Check sheet for the modelled part. Datum: model origin and axes. Units: mm. A direction names the side the tool comes from. Round coordinates to 2 decimals unless told otherwise and drop trailing zeros. Write each loop counter-clockwise with the first axis right and the second up, starting at its lowest first coordinate (ties: lowest second). Pieces come first, ordered by that corner, then holes. Notation, with made-up numbers: (-39, -22) - (3, -22) arc R11 ccw to (3, -2) - close; hole circle Ø2 at (35, 26.25). An arc over 180 degrees is marked (long way). Answer as a JSON object with one key per item and string values. Group by question number.
Item 1: Thickness scan on line 1 (Y direction, x = -0.5, z = 13); line 2 (Y direction, x = 31, z = 14.5); line 3 (Y direction, x = 42, z = 2). Record the ranges inside material, lowest first.
Item 2: Sectioned sample at B-B on z = 13.75. Count the separate pieces of the cut face and the enclosed holes in it, plus the area to 3 significant figures.
Item 3: Gauge pin test, flat ends, axial feed: P1, Ø1, axis at y = 29.5, z = 12, coming from the +X side; P2, Ø0.6, axis at x = 16, y = 10.5, coming from the +Z side; P3, Ø4, axis at x = 15.5, y = 42.5, coming from the +Z side. Record the tip position at first contact, or that the pin passes through.
Item 4: Sectioned sample at C-C on x = 3.5. Record the boundary of the cut face in (y, z), plus the area to 3 significant figures.
Item 5: Set-up check for faces 1 (the flat face through (-6, 42.249, 7)), 2 (the flat face through (35, 46.247, 10)), 3 (the flat face through (17.1, 18.4, 2)): record each of +Z, -Z, +X, -X, +Y, -Y from which the full face is reachable in a straight line by a thin tool's end or side.
Item 6: Release check for a two-part mould opening along Y. For faces 4 (the flat face through (16, 62.251, 8)), 5 (the flat face through (-2, -1.747, 10)), 6 (the flat face through (12.48, 21.47, 1.97)), 7 (the flat face through (-13.672, -8, 8)) record: pulls with the +Y half, pulls with the -Y half, needs draft (parallel to the pull), parting line crosses it, or undercut.
Item 7: Sectioned sample at D-D on y = 56.5. Record the boundary of the cut face in (x, z).
Item 8: Sectioned sample at A-A on x = 37.5. Record the boundary of the cut face in (y, z).
```python
from build123d import *

# Parameters (mm, degrees)
SKETCH1_W           = 60.000998497
SKETCH1_H           = 80.001998902
BOSS_EXTRUDE1_DEPTH = 15.001
SKETCH2_W           = 14.999998093
SKETCH2_H           = 39.998000621
CUT_EXTRUDE1_DEPTH  = 80.035391071
SKETCH3_W           = 14.99999988
SKETCH3_H           = 39.998000621
CUT_EXTRUDE2_DEPTH  = 80.035391071
CUT_EXTRUDE3_DEPTH  = 11.003000021
BOSS_EXTRUDE2_DEPTH = 6.004000425
CUT_EXTRUDE4_DEPTH  = 80.035391071
CUT_EXTRUDE5_DEPTH  = 80.035391071
BOSS_EXTRUDE3_DEPTH = 6.004000425
CUT_EXTRUDE6_DEPTH  = 80.035391071
BOSS_EXTRUDE4_DEPTH = 11.003000021
CUT_EXTRUDE7_DEPTH  = 11.003000021
BOSS_EXTRUDE5_DEPTH = 11.003000021
CUT_EXTRUDE8_DEPTH  = 11.003000021


with BuildPart() as part:
    # Sketch1 → Boss-Extrude1 (new body)
    with BuildSketch(Plane.XY.offset(15)):
        with Locations((16.328499318, 22.25)):
            Rectangle(SKETCH1_W, SKETCH1_H)
    extrude(amount=-BOSS_EXTRUDE1_DEPTH)

    # Sketch2 → Cut-Extrude1 (cut, through all)
    with BuildSketch(Plane(origin=(0, 0, -0.001), x_dir=(-1, 0, 0), z_dir=(0, 0, -1))):
        with Locations((-38.82899952, 22.250000239)):
            Rectangle(SKETCH2_W, SKETCH2_H)
    extrude(amount=-CUT_EXTRUDE1_DEPTH, mode=Mode.SUBTRACT)

    # Sketch3 → Cut-Extrude2 (cut, through all)
    with BuildSketch(Plane(origin=(0, 0, -0.001), x_dir=(-1, 0, 0), z_dir=(0, 0, -1))):
        with Locations((6.171999991, 22.250000239)):
            Rectangle(SKETCH3_W, SKETCH3_H)
    extrude(amount=-CUT_EXTRUDE2_DEPTH, mode=Mode.SUBTRACT)

    # Sketch4 → Cut-Extrude3 (cut)
    with BuildSketch(Plane.XY.offset(15)):
        Polygon((27.332000732, 42.25), (27.332000732, 46.247001648), (42.331001282, 46.247001648), (42.331001282, 58.252998352), (-9.673999786, 58.252998352), (-9.673999786, 46.247001648), (5.324999809, 46.247001648), (5.324999809, 42.25), (5.326000214, 42.25), (5.326000214, 2.249000072), (5.324999809, 2.249000072), (5.324999809, -1.746999979), (-9.673999786, -1.746999979), (-9.673999786, -13.753000259), (42.331001282, -13.753000259), (42.331001282, -1.746999979), (27.332000732, -1.746999979), (27.332000732, 2.249000072), (27.330999374, 2.249000072), (27.330999374, 42.25), align=None)
    extrude(amount=-CUT_EXTRUDE3_DEPTH, mode=Mode.SUBTRACT)

    # Sketch5 → Boss-Extrude2 (add)
    with BuildSketch(Plane.XY.offset(3.996999979)):
        Polygon((16.327999115, 4.750999928), (17.579000473, 4.414999962), (18.493999481, 3.5), (18.829000473, 2.25), (18.493999481, 1), (17.579000473, 0.085000001), (16.327999115, -0.25), (15.078000069, 0.085000001), (14.163000107, 1), (13.828000069, 2.25), (14.163000107, 3.5), (15.078000069, 4.414999962), align=None)
    extrude(amount=BOSS_EXTRUDE2_DEPTH)

    # Sketch6 → Cut-Extrude4 (cut, through all)
    with BuildSketch(Plane(origin=(0, 0, -0.001), x_dir=(-1, 0, 0), z_dir=(0, 0, -1))):
        Polygon((-16.829999924, 3.114000082), (-17.197000504, 2.747999907), (-17.330999374, 2.247999907), (-17.197000504, 1.746999979), (-16.829999924, 1.381000042), (-16.327999115, 1.246999979), (-15.826999664, 1.381000042), (-15.460000038, 1.746999979), (-15.324999809, 2.247999907), (-15.460000038, 2.747999907), (-15.826999664, 3.114000082), (-16.327999115, 3.247999907), align=None)
    extrude(amount=-CUT_EXTRUDE4_DEPTH, mode=Mode.SUBTRACT)

    # Sketch7 → Cut-Extrude5 (cut, through all)
    with BuildSketch(Plane(origin=(0, 0, -0.001), x_dir=(-1, 0, 0), z_dir=(0, 0, -1))):
        Polygon((-13.498000145, 19.419000626), (-12.630000114, 20.718000412), (-12.324999809, 22.25), (-12.630000114, 23.781999588), (-13.498000145, 25.080999374), (-14.796999931, 25.947999954), (-16.327999115, 26.253000259), (-17.86000061, 25.947999954), (-19.159000397, 25.080999374), (-20.027000427, 23.781999588), (-20.330999374, 22.25), (-20.027000427, 20.718000412), (-19.159000397, 19.419000626), (-17.86000061, 18.552000046), (-16.327999115, 18.246999741), (-14.796999931, 18.552000046), align=None)
    extrude(amount=-CUT_EXTRUDE5_DEPTH, mode=Mode.SUBTRACT)

    # Sketch8 → Boss-Extrude3 (add)
    with BuildSketch(Plane.XY.offset(3.996999979)):
        Polygon((15.078000069, 40.084999084), (14.163000107, 41), (13.828000069, 42.25), (14.163000107, 43.5), (15.078000069, 44.415000916), (16.327999115, 44.750999451), (17.579000473, 44.415000916), (18.493999481, 43.5), (18.829000473, 42.25), (18.493999481, 41), (17.579000473, 40.084999084), (16.327999115, 39.75), align=None)
    extrude(amount=BOSS_EXTRUDE3_DEPTH)

    # Sketch9 → Cut-Extrude6 (cut, through all)
    with BuildSketch(Plane(origin=(0, 0, -0.001), x_dir=(-1, 0, 0), z_dir=(0, 0, -1))):
        Polygon((-15.826999664, 41.386001587), (-15.460000038, 41.751998901), (-15.324999809, 42.251998901), (-15.460000038, 42.752998352), (-15.826999664, 43.118999481), (-16.327999115, 43.252998352), (-16.829999924, 43.118999481), (-17.197000504, 42.752998352), (-17.330999374, 42.251998901), (-17.197000504, 41.751998901), (-16.829999924, 41.386001587), (-16.327999115, 41.251998901), align=None)
    extrude(amount=-CUT_EXTRUDE6_DEPTH, mode=Mode.SUBTRACT)

    # Sketch10 → Boss-Extrude4 (add)
    with BuildSketch(Plane.XY.offset(3.996999979)):
        Polygon((14.163000107, 9), (13.828000069, 10.25), (14.163000107, 11.5), (15.078000069, 12.414999962), (16.327999115, 12.75), (17.579000473, 12.414999962), (18.493999481, 11.5), (18.829000473, 10.25), (18.493999481, 9), (17.579000473, 8.085000038), (16.327999115, 7.75), (15.078000069, 8.085000038), align=None)
    extrude(amount=BOSS_EXTRUDE4_DEPTH)

    # Sketch11 → Cut-Extrude7 (cut)
    with BuildSketch(Plane.XY.offset(15)):
        Polygon((16.829999924, 9.380999565), (17.197000504, 9.748000145), (17.330999374, 10.25), (17.197000504, 10.751999855), (16.829999924, 11.119000435), (16.327999115, 11.253000259), (15.826999664, 11.119000435), (15.460000038, 10.751999855), (15.324999809, 10.25), (15.460000038, 9.748000145), (15.826999664, 9.380999565), (16.327999115, 9.246999741), align=None)
    extrude(amount=-CUT_EXTRUDE7_DEPTH, mode=Mode.SUBTRACT)

    # Sketch12 → Boss-Extrude5 (add)
    with BuildSketch(Plane.XY.offset(3.996999979)):
        Polygon((17.579000473, 36.415000916), (18.493999481, 35.5), (18.829000473, 34.25), (18.493999481, 33), (17.579000473, 32.084999084), (16.327999115, 31.75), (15.078000069, 32.084999084), (14.163000107, 33), (13.828000069, 34.25), (14.163000107, 35.5), (15.078000069, 36.415000916), (16.327999115, 36.750999451), align=None)
    extrude(amount=BOSS_EXTRUDE5_DEPTH)

    # Sketch13 → Cut-Extrude8 (cut)
    with BuildSketch(Plane.XY.offset(15)):
        Polygon((15.826999664, 35.118999481), (15.460000038, 34.751998901), (15.324999809, 34.25), (15.460000038, 33.748001099), (15.826999664, 33.381000519), (16.327999115, 33.247001648), (16.829999924, 33.381000519), (17.197000504, 33.748001099), (17.330999374, 34.25), (17.197000504, 34.751998901), (16.829999924, 35.118999481), (16.327999115, 35.252998352), align=None)
    extrude(amount=-CUT_EXTRUDE8_DEPTH, mode=Mode.SUBTRACT)


solid = part.part
```
Completed:
{
 "1": {"line 1": "-17.75 to -13.75, -1.75 to 2.25, 42.25 to 46.25, 58.25 to 62.25", "line 2": "-17.75 to -13.75, -1.75 to 46.25, 58.25 to 62.25", "line 3": "-17.75 to 2.25, 42.25 to 62.25"},
 "2": {"separate pieces": "3", "enclosed holes": "3", "area": "1,330 mm²"},
 "3": {"P1": "x = 31.33", "P2": "z = 4", "P3": "z = 10"},
 "4": {"outline": "(-17.75, 0) - (62.25, 0) - (62.25, 15) - (58.25, 15) - (58.25, 4) - (46.25, 4) - (46.25, 15) - (-1.75, 15) - (-1.75, 4) - (-13.75, 4) - (-13.75, 15) - (-17.75, 15) - close", "area": "936 mm²"},
 "5": {"face 1": "+Z, -Z, -X", "face 2": "+Z", "face 3": "+Z, -Z"},
 "6": {"face 4": "pulls with the +Y half", "face 5": "undercut", "face 6": "undercut", "face 7": "needs draft"},
 "7": {"outline": "(-13.67, 0) - (46.33, 0) - (46.33, 15) - (42.33, 15) - (42.33, 4) - (-9.67, 4) - (-9.67, 15) - (-13.67, 15) - close"},
 "8": {"outline": "(-17.75, 0) - (2.25, 0) - (2.25, 15) - (-1.75, 15) - (-1.75, 4) - (-13.75, 4) - (-13.75, 15) - (-17.75, 15) - close; (42.25, 0) - (62.25, 0) - (62.25, 15) - (58.25, 15) - (58.25, 4) - (46.25, 4) - (46.25, 15) - (42.25, 15) - close"}
}
